from build123d import *

# Parameters (mm, degrees)
SKETCH1_R                   = 10.668
EXTRUDE1_DEPTH              = 12.7
SKETCH2_R                   = 6.858
CUT_EXTRUDE1_DEPTH          = 10.20572
CUT_EXTRUDE1_DRAFT          = -1.783333333
SKETCH5_R                   = 7.563555556
CUT_EXTRUDE3_DEPTH          = 3.175
CUT_EXTRUDE3_DRAFT          = -45
CIRPATTERN1_COPY_1_SKETCH_R = 6.858
CIRPATTERN1_COPY_1_DEPTH    = 10.20572
CIRPATTERN1_COPY_1_DRAFT    = -1.783333333
CIRPATTERN1_COPY_2_SKETCH_R = 7.563555556
CIRPATTERN1_COPY_2_DEPTH    = 3.175
CIRPATTERN1_COPY_2_DRAFT    = -45
FILLET1_R                   = 0.381


with BuildPart() as part:
    # Sketch1 → Extrude1 (new, symmetric)
    with BuildSketch(Plane.XY):
        Circle(SKETCH1_R)
    extrude(amount=EXTRUDE1_DEPTH, both=True)


with BuildPart() as cut_extrude1_tool:
    # Sketch2 → Cut-Extrude1 (with draft: the straight prism first)
    with BuildSketch(Plane.XY.offset(12.7)):
        Circle(SKETCH2_R)
    extrude(amount=-CUT_EXTRUDE1_DEPTH)
    # Cut-Extrude1: the draft: its side faces are tilted about the plane it starts from
    cut_extrude1_sides = [cut_extrude1_tool.faces().sort_by_distance(p)[0] for p in [
        (-6.858, 0, 7.59714),
    ]]
    draft(cut_extrude1_sides, Plane.XY.offset(12.7), CUT_EXTRUDE1_DRAFT)


with BuildPart() as part_1:
    add(part.part)

    # Cut-Extrude1: cut by cut_extrude1_tool
    add(cut_extrude1_tool.part, mode=Mode.SUBTRACT)


with BuildPart() as cut_extrude3_tool:
    # Sketch5 → Cut-Extrude3 (with draft: the straight prism first)
    with BuildSketch(Plane.XY.offset(12.7)):
        Circle(SKETCH5_R)
    extrude(amount=-CUT_EXTRUDE3_DEPTH)
    # Cut-Extrude3: the draft: its side faces are tilted about the plane it starts from
    cut_extrude3_sides = [cut_extrude3_tool.faces().sort_by_distance(p)[0] for p in [
        (-7.563555556, 0, 11.1125),
    ]]
    draft(cut_extrude3_sides, Plane.XY.offset(12.7), CUT_EXTRUDE3_DRAFT)


with BuildPart() as part_2:
    add(part_1.part)

    # Cut-Extrude3: cut by cut_extrude3_tool
    add(cut_extrude3_tool.part, mode=Mode.SUBTRACT)


with BuildPart() as cirpattern1_copy_1_tool:
    # CirPattern1 copy 1 sketch → CirPattern1 copy 1 (with draft: the straight prism first)
    with BuildSketch(Plane(origin=(0, 0, -12.7), x_dir=(-1, 0, 0), z_dir=(0, 0, -1))):
        Circle(CIRPATTERN1_COPY_1_SKETCH_R)
    extrude(amount=-CIRPATTERN1_COPY_1_DEPTH)
    # CirPattern1 copy 1: the draft: its side faces are tilted about the plane it starts from
    cirpattern1_copy_1_sides = [cirpattern1_copy_1_tool.faces().sort_by_distance(p)[0] for p in [
        (6.858, 0, -7.59714),
    ]]
    draft(cirpattern1_copy_1_sides, Plane(origin=(0, 0, -12.7), x_dir=(-1, 0, 0), z_dir=(0, 0, -1)), CIRPATTERN1_COPY_1_DRAFT)


with BuildPart() as part_3:
    add(part_2.part)

    # CirPattern1 copy 1: cut by cirpattern1_copy_1_tool
    add(cirpattern1_copy_1_tool.part, mode=Mode.SUBTRACT)


with BuildPart() as cirpattern1_copy_2_tool:
    # CirPattern1 copy 2 sketch → CirPattern1 copy 2 (with draft: the straight prism first)
    with BuildSketch(Plane(origin=(0, 0, -12.7), x_dir=(-1, 0, 0), z_dir=(0, 0, -1))):
        Circle(CIRPATTERN1_COPY_2_SKETCH_R)
    extrude(amount=-CIRPATTERN1_COPY_2_DEPTH)
    # CirPattern1 copy 2: the draft: its side faces are tilted about the plane it starts from
    cirpattern1_copy_2_sides = [cirpattern1_copy_2_tool.faces().sort_by_distance(p)[0] for p in [
        (7.563555556, 0, -11.1125),
    ]]
    draft(cirpattern1_copy_2_sides, Plane(origin=(0, 0, -12.7), x_dir=(-1, 0, 0), z_dir=(0, 0, -1)), CIRPATTERN1_COPY_2_DRAFT)


with BuildPart() as part_4:
    add(part_3.part)

    # CirPattern1 copy 2: cut by cirpattern1_copy_2_tool
    add(cirpattern1_copy_2_tool.part, mode=Mode.SUBTRACT)

    # Fillet1
    fillet1_edges = [part_4.edges().sort_by_distance(p)[0] for p in [
        (-10.668, 0, -12.7),
        (-10.668, 0, 12.7),
    ]]
    fillet(fillet1_edges, radius=FILLET1_R)


solid = part_4.part
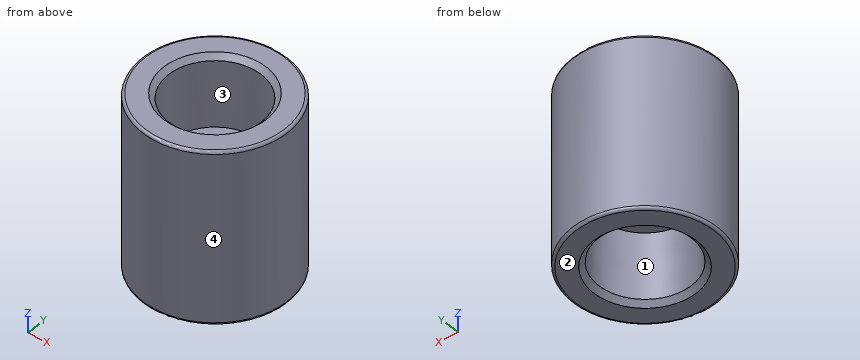
Here's how the part is built. I have some questions about the finished solid (model axes, mm). Face numbers are marked on the shaded views. Round coordinates to 2 decimals unless told otherwise and drop trailing zeros. Order: outer loops, then holes, each group sorted by start corner. A loop starts at its lowest first (then second) coordinate and runs counter-clockwise, first axis right, second up. Notation, with made-up numbers: M 67,-1 L 121,-1 A24 ccw 121,12 Z; hole C 35.5,3 d4. An arc over 180 degrees is marked long. One line per question, with ' | ' between items.
1) We'd pull the mould along Y, two halves only. Please class the marked faces 1, 2, 3 and 4: released by +Y, released by -Y, zero draft, split by the parting line, or undercut.
Checked values:
face 1: undercut | face 2: zero draft | face 3: undercut | face 4: split by the parting line
2) I'm going to push flat-ended pins straight in: pin 1 Ø6.5 at (x, y) = (-2.5, -3) entering from -Z; pin 2 Ø1.5 at (x, z) = (7, -9.5) entering from +Y; pin 3 Ø1 at (y, z) = (5, -4) entering from -X. Where does each tip first touch, or does it pass through?
Checked values:
pin 1: stops at z = -12.29 | pin 2: stops at y = 8.65 | pin 3: stops at x = -9.67
3) Imagine slicing it at C-C, the plane z = 3.5. Write out the boundary of the cut face in (x, y).
Checked values:
outline: C 0,0 d21.34; hole C 0,0 d13.14
4) Imagine slicing it at A-A, the plane x = 0. Write out the boundary of the cut face in (y, z).
Checked values:
outline: M -10.67,-12.32 A0.38 ccw -10.29,-12.7 L -7.56,-12.7 L -6.84,-11.97 L -6.54,-2.49 L 6.54,-2.49 L 6.84,-11.97 L 7.56,-12.7 L 10.29,-12.7 A0.38 ccw 10.67,-12.32 L 10.67,12.32 A0.38 ccw 10.29,12.7 L 7.56,12.7 L 6.84,11.97 L 6.54,2.49 L -6.54,2.49 L -6.84,11.97 L -7.56,12.7 L -10.29,12.7 A0.38 ccw -10.67,12.32 Z
5) I need wall thicknesses on line 1 (Z direction, x = -5, y = 0.5); line 2 (Y direction, x = -5.5, z = 4); line 3 (Y direction, x = 3.5, z = -7.25). Which ranges of each line are inside material? Lowest first, please.
Checked values:
line 1: z = -2.49 to 2.49 | line 2: y = -9.14 to -3.62, 3.62 to 9.14 | line 3: y = -10.08 to -5.7, 5.7 to 10.08
6) Imagine slicing it at D-D, the plane z = -10.75. Write out the boundary of the cut face in (x, y).
Checked values:
outline: C 0,0 d21.34; hole C 0,0 d13.59
